Geometry: see drawing. Coordinates: mm, zero at the bounding-box minimum. A direction names the side the tool comes from. Coordinates: 2 decimals unless noted, no trailing zeros. Loops run counter-clockwise (first coordinate to the right, second up) from the corner with the lowest first, then second, coordinate; pieces in that order, holes last. Notation, with made-up numbers: (25, 37.5) -> (68, 37.5) arc R19 cw to (68, 73.5) -> close; hole circle Ø8 at (-18.5, 62). An arc over 180 degrees is marked (long way). Put each result on its own line as item: value. Start each with the question number.
1) Cut plane C-C (x = 159). Return the cut outline in (y, z).
2) Material intervals for L1, parallel to X at y = 22.5, z = 199; L2, parallel to Z at x = 321, y = 73; L3, parallel to Y at x = 31.5, z = 173, sorted ascending.
3) Cut plane A-A (z = 56.5). Return the cut outline in (x, y), plus the area to 3 significant figures.
4) Contact query for a flat-ended pin moving along its axis: P1, Ø2, axis at x = 288.5, z = 209.5, coming from the +Y side. Output: stop coordinate, or through.
5) Pull-direction query (X, two-part tool) for the marked faces 3, 4, 5 and 6; classes: pulls with the +X half, pulls with the -X half, needs draft (parallel to the pull), parting line crosses it, or undercut.
6) Cut plane B-B (y = 79). Return the cut outline in (x, z).
7) Set-up query: the marked faces 1 and 2. Return all of +Z, -Z, +X, -X, +Y, -Y with unobstructed straight access to the full face (end or side cutting, diameter ignored); none if empty.
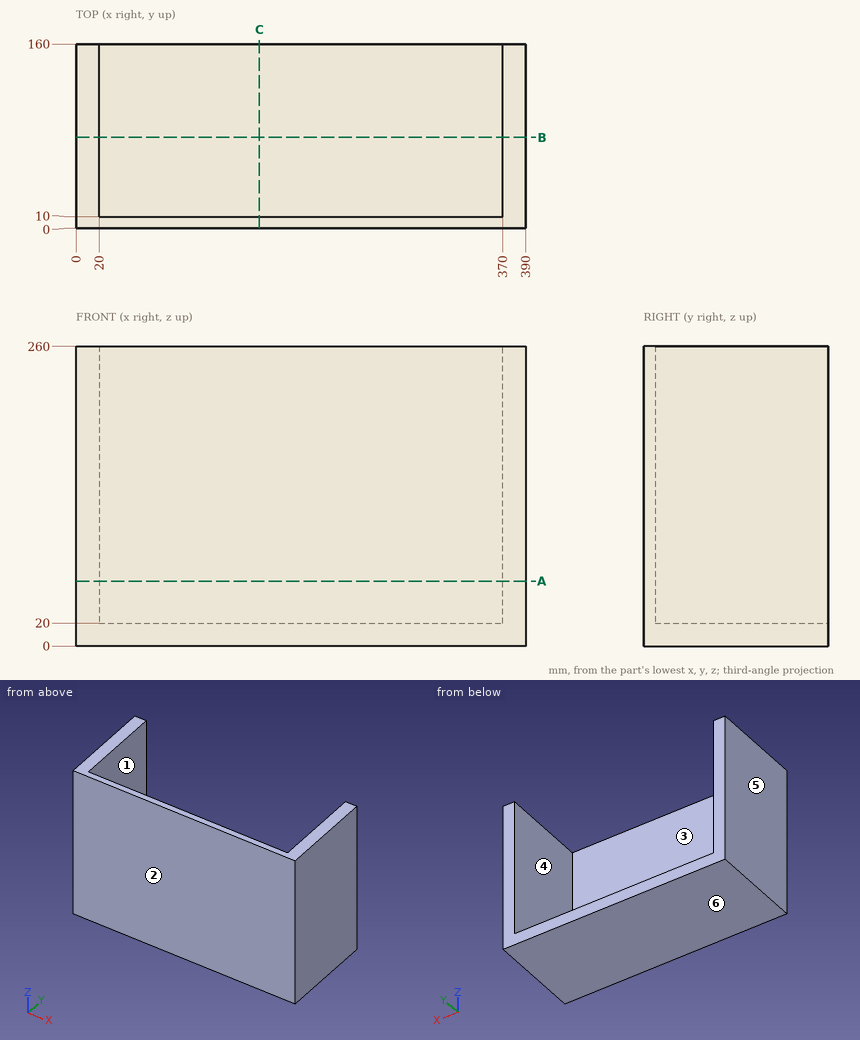
Results found:
1. outline: (0, 0) -> (160, 0) -> (160, 20) -> (10, 20) -> (10, 260) -> (0, 260) -> close
2. L1: x = 0 to 20, 370 to 390
2. L2: z = 0 to 20
2. L3: y = 0 to 10
3. outline: (0, 0) -> (390, 0) -> (390, 160) -> (370, 160) -> (370, 10) -> (20, 10) -> (20, 160) -> (0, 160) -> close
3. area: 9,900 mm2
4. P1: stops at y = 10
5. face 3: undercut
5. face 4: undercut
5. face 5: pulls with the -X half
5. face 6: needs draft
6. outline: (0, 0) -> (390, 0) -> (390, 260) -> (370, 260) -> (370, 20) -> (20, 20) -> (20, 260) -> (0, 260) -> close
7. face 1: +Z, +Y
7. face 2: +Z, -Z, +X, -X, -Y
